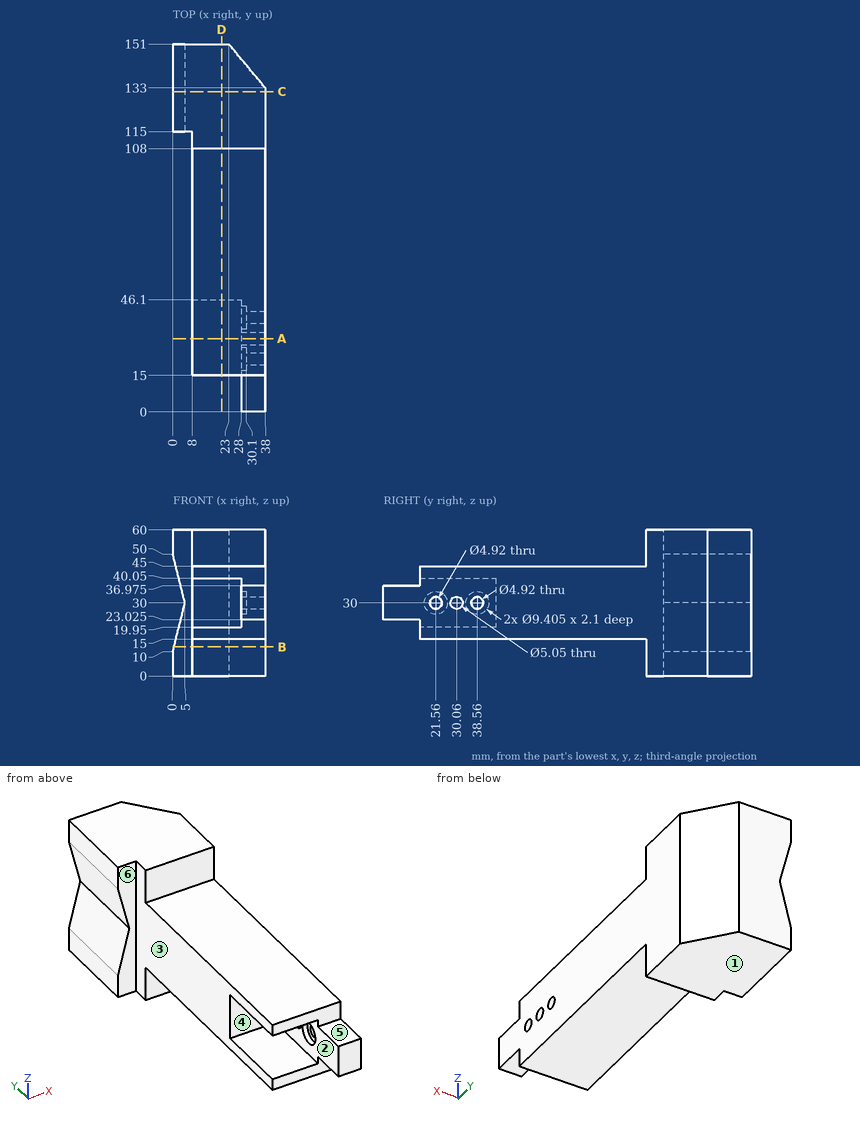
Here's the drawing with two shaded views (mm, measured from the low corner). I have some questions. A direction names the side the tool comes from. Round coordinates to 2 decimals unless told otherwise and drop trailing zeros. Loops run counter-clockwise (first coordinate to the right, second up) from the corner with the lowest first, then second, coordinate; pieces in that order, holes last. Notation, with made-up numbers: M 20.5,60 L 55.5,60 A30 ccw 55.5,91 Z; hole C 5.25,46.5 d7. An arc over 180 degrees is marked long. Answer as a JSON object with one key per item and string values. Group by question number.
Q1. Imagine slicing it at A-A, the plane y = 30.06. Please give me the cut outline in (x, z) (3 decimals), then the cut area to 4 significant figures.
Q2. Please list where these lines run through material, in increasing order: L1, parallel to Y at x = 29, z = 30 (1 decimal); L2, parallel to Z at x = 29, y = 21; L3, parallel to Y at x = 30, z = 30 (1 decimal).
Q3. Will these pins go through, and if not, where does the flat tip stop? pin 1 (4.5 mm diameter, centred on y = 30.06, z = 30, fed in from -X); pin 2 (4.5 mm diameter, centred on x = 23.5, z = 6, fed in from -Y); pin 3 (8.5 mm diameter, centred on y = 38.56, z = 30, fed in from -X); pin 4 (16 mm diameter, centred on x = 14, z = 31, fed in from -Y).
Q4. Imagine slicing it at D-D, the plane x = 20. Please give me the cut outline in (y, z).
Q5. On a 3-axis mill with a long thin cutter (end or side, diameter ignored), from which of +Z, -Z, +X, -X, +Y, -Y can I reach the whole of each face in a straight line? I mean the marked faces 4, 5 and 6. Say none if no direction works.
Q6. Imagine slicing it at B-B, the plane z = 12. Please give me the cut outline in (x, y), then the cut area to 4 significant figures.
Q7. We'd pull the mould along Z, two halves only. Please class the marked faces 1, 2 and 3: +Z half, -Z half, draft (parallel to the pull), parting line (faces both ways), or undercut.
Q8. Imagine slicing it at C-C, the plane y = 131.5. Please give me the cut outline in (x, z).
Findings:
{
 "1": {"outline": "M 8,15 L 38,15 L 38,27.475 L 28,27.475 L 28,19.95 L 8,19.95 Z; M 8,40.05 L 28,40.05 L 28,32.525 L 38,32.525 L 38,45 L 8,45 Z", "area": "447.5 mm2"},
 "2": {"L1": "y = 0 to 16.9, 26.3 to 27.5, 32.6 to 33.9, 43.3 to 143.8", "L2": "z = 15 to 25.33, 34.67 to 45", "L3": "y = 0 to 16.9, 26.3 to 27.5, 32.6 to 33.9, 43.3 to 142.6"},
 "3": {"pin 1": "passes through", "pin 2": "stops at y = 108", "pin 3": "stops at x = 30.1", "pin 4": "stops at y = 46.1"},
 "4": {"outline": "M 15,15 L 108,15 L 108,0 L 151,0 L 151,60 L 108,60 L 108,45 L 15,45 L 15,40.05 L 46.1,40.05 L 46.1,19.95 L 15,19.95 Z"},
 "5": {"face 4": "-X, -Y", "face 5": "+Z, +X, -X, -Y", "face 6": "+Z, -Z, -X, -Y"},
 "6": {"outline": "M 0.5,115 L 8,115 L 8,108 L 38,108 L 38,133 L 23,151 L 0.5,151 Z", "area": "1,425 mm2"},
 "7": {"face 1": "-Z half", "face 2": "undercut", "face 3": "draft"},
 "8": {"outline": "M 0,0 L 38,0 L 38,60 L 0,60 L 0,50 L 5,30 L 0,10 Z"}
}
